from build123d import *

# Parameters (mm, degrees)
SKETCH10_W           = 35
SKETCH10_H           = 26
BOSS_EXTRUDE4_DEPTH  = 2.5
SKETCH1_R            = 1.5
BOSS_EXTRUDE5_DEPTH  = 5
SKETCH11_W           = 35
SKETCH11_H           = 26
BOSS_EXTRUDE6_DEPTH  = 2.5
CUT_EXTRUDE1_START   = -13
CUT_EXTRUDE1_DEPTH   = 56.676105727
SKETCH4_R            = 7.6
CUT_EXTRUDE2_DEPTH   = 1.2
SKETCH5_R            = 6.6
CUT_EXTRUDE3_DEPTH   = 50.27874954
SKETCH12_W           = 35
SKETCH12_H           = 26
BOSS_EXTRUDE7_DEPTH  = 15
SKETCH13_W           = 35
SKETCH13_H           = 26
BOSS_EXTRUDE8_DEPTH  = 7.5
SKETCH14_R           = 1.5
BOSS_EXTRUDE9_DEPTH  = 5
SKETCH15_W           = 35
SKETCH15_H           = 26
BOSS_EXTRUDE10_DEPTH = 2.5
SKETCH8_R            = 4
CUT_EXTRUDE6_DEPTH   = 62.021677757
FILLET1_R            = 13


with BuildPart() as part:
    # Sketch10 → Boss-Extrude4 (new body)
    with BuildSketch(Plane(origin=(0, 0, 0), x_dir=(1, 0, 0), z_dir=(0, 1, 0))):
        with Locations((15.5, -23)):
            Rectangle(SKETCH10_W, SKETCH10_H)
    extrude(amount=BOSS_EXTRUDE4_DEPTH)

    # Sketch1 → Boss-Extrude5 (add)
    with BuildSketch(Plane(origin=(0, 0, 0), x_dir=(1, 0, 0), z_dir=(0, 1, 0))):
        Polygon((0, 0), (6, 0), (6, -10), (25, -10), (25, 0), (31, 0), (31, -10), (33, -10), (33, -36), (-2, -36), (-2, -10), (0, -10), align=None)
        with Locations(Location((3, -5, 0), (0, 0, 270))):
            Circle(SKETCH1_R, mode=Mode.SUBTRACT)
        with Locations(Location((28, -5, 0), (0, 0, 90))):
            Circle(SKETCH1_R, mode=Mode.SUBTRACT)
    extrude(amount=-BOSS_EXTRUDE5_DEPTH)

    # Sketch11 → Boss-Extrude6 (add)
    with BuildSketch(Plane.XZ.offset(5)):
        with Locations((15.5, 23)):
            Rectangle(SKETCH11_W, SKETCH11_H)
    extrude(amount=BOSS_EXTRUDE6_DEPTH)

    # Sketch3 → Cut-Extrude1 (cut)
    with BuildSketch(Plane(origin=(0, 0, 10), x_dir=(-1, 0, 0), z_dir=(0, 0, -1)).offset(CUT_EXTRUDE1_START)):
        Polygon((-22.1, 2.5), (-22.1, 0.2875), (-23.1, 0.2875), (-23.1, -0.9125), (-15.5, -0.9125), (-7.9, -0.9125), (-7.9, 0.2875), (-8.9, 0.2875), (-8.9, 2.5), align=None)
    cut_extrude1 = extrude(amount=CUT_EXTRUDE1_DEPTH, mode=Mode.SUBTRACT)

    # Sketch4 → Cut-Extrude2 (cut)
    with BuildSketch(Plane(origin=(0, -0.9125, 0), x_dir=(1, 0, 0), z_dir=(0, 1, 0))):
        with Locations((15.5, -23)):
            Circle(SKETCH4_R)
    cut_extrude2 = extrude(amount=CUT_EXTRUDE2_DEPTH, mode=Mode.SUBTRACT)

    # Sketch5 → Cut-Extrude3 (cut, through all)
    with BuildSketch(Plane(origin=(0, -0.9125, 0), x_dir=(1, 0, 0), z_dir=(0, 1, 0))):
        with Locations((15.5, -23)):
            Circle(SKETCH5_R)
    cut_extrude3 = extrude(amount=CUT_EXTRUDE3_DEPTH, mode=Mode.SUBTRACT)

    # Sketch12 → Boss-Extrude7 (add)
    with BuildSketch(Plane.XZ.offset(7.5)):
        with Locations((15.5, 23)):
            Rectangle(SKETCH12_W, SKETCH12_H)
    extrude(amount=BOSS_EXTRUDE7_DEPTH)

    # Sketch13 → Boss-Extrude8 (add)
    with BuildSketch(Plane.XZ.offset(22.5)):
        with Locations((15.5, 23)):
            Rectangle(SKETCH13_W, SKETCH13_H)
    extrude(amount=BOSS_EXTRUDE8_DEPTH)

    # Sketch14 → Boss-Extrude9 (add)
    with BuildSketch(Plane.XZ.offset(30)):
        Polygon((0, 0), (6, 0), (6, 10), (25, 10), (25, 0), (31, 0), (31, 10), (33, 10), (33, 36), (-2, 36), (-2, 10), (0, 10), align=None)
        with Locations(Location((3, 5, 0), (0, 0, 90))):
            Circle(SKETCH14_R, mode=Mode.SUBTRACT)
        with Locations(Location((28, 5, 0), (0, 0, 270))):
            Circle(SKETCH14_R, mode=Mode.SUBTRACT)
    extrude(amount=BOSS_EXTRUDE9_DEPTH)

    # Sketch15 → Boss-Extrude10 (add)
    with BuildSketch(Plane.XZ.offset(35)):
        with Locations((15.5, 23)):
            Rectangle(SKETCH15_W, SKETCH15_H)
    extrude(amount=BOSS_EXTRUDE10_DEPTH)

    # Mirror8: Cut-Extrude1, Cut-Extrude2, Cut-Extrude3 across plane
    add(cut_extrude1.mirror(Plane.ZX.offset(-17.5)), mode=Mode.SUBTRACT)
    add(cut_extrude2.mirror(Plane.ZX.offset(-17.5)), mode=Mode.SUBTRACT)
    add(cut_extrude3.mirror(Plane.ZX.offset(-17.5)), mode=Mode.SUBTRACT)

    # Sketch8 → Cut-Extrude6 (cut, through all)
    with BuildSketch(Plane(origin=(0, -0.9125, 0), x_dir=(1, 0, 0), z_dir=(0, 1, 0))):
        with Locations(Location((15.5, -23, 0), (0, 0, 270))):
            Circle(SKETCH8_R)
    extrude(amount=-CUT_EXTRUDE6_DEPTH, mode=Mode.SUBTRACT)

    # Fillet1
    fillet1_edges = [part.edges().sort_by_distance(p)[0] for p in [
        (33, -17.5, 36),
        (-2, -17.5, 36),
    ]]
    fillet(fillet1_edges, radius=FILLET1_R)


solid = part.part
Design review of the part built by this model. Coordinates are the model's own, in mm. A direction names the side the tool comes from. Give positions to 0.01 mm unless a question says otherwise; leave off trailing zeros. Loops run counter-clockwise (first coordinate to the right, second up) from the corner with the lowest first, then second, coordinate; pieces in that order, holes last. Notation, with made-up numbers: (-1.5, 1.5) - (22.5, 1.5) arc R21 ccw to (22.5, 38.5) - close; hole circle Ø8 at (48.25, 56). An arc over 180 degrees is marked (long way). Use CSV: the item, a comma, the result in double quotes. Start each with the question number.
1. Wall thickness on L1, parallel to X at y = -32.15, z = 5; L2, parallel to Y at x = 23, z = 18; L3, parallel to X at y = 1, z = 17.5: over which ranges is each line inside the solid? List them lowest first.
2. Add section D-D (y = -8.5). State the section outline as (x, z) points, plus the area to 3 significant figures.
3. Machinability: for faces 5 (the flat face through (22.1, -36, 17)), 6 (the flat face through (25, -32, 5)), 7 (the flat face through (4.4, 0, 6)), which of the approach directions +Z, -Z, +X, -X, +Y, -Y give a long, thin tool a straight path to every point of the face, cutting with its end or side? Answer none if there is none.
4. Add section A-A (x = 15.5). State the section outline as (y, z) points, plus the area to 3 significant figures.
5. Add section B-B (z = 5). Count the separate pieces of the cut face and the enclosed holes in it, plus the area to 3 significant figures.
6. Add section C-C (y = -33). State the section outline as (x, z) points.
7. Draft analysis for pull direction Y (two halves, no side actions). For faces 1 (the flat face through (11, -37.5, 29)), 2 (the cylindrical face through (15.4, -36.4, 29.6)), 3 (the cylindrical face through (15.33, -0.32, 30.6)), 4 (the flat face through (8.7, -35.288, 21.1)), state which applies: released by +Y, released by -Y, zero draft, split by the parting line, or undercut.
8. Insertion check: P1, Ø3, axis at x = 3.5, y = -25.5, coming from the -Z side; P2, Ø4.5, axis at x = 17.5, z = 22, coming from the -Y side; P3, Ø12, axis at y = -26.5, z = 26.5, coming from the +X side; P4, Ø6.5, axis at x = 4.5, z = 5, coming from the +Y side. Each pin has a flat end and moves straight along its axis. Give the tip position at first contact, or say it passes through.
Results found:
1,L1,"x = 0 to 1.5, 4.5 to 6, 25 to 26.5, 29.5 to 31"
1,L2,"y = -37.5 to -35.29, -34.09 to -0.91, 0.29 to 2.5"
1,L3,"x = -2 to 8.9, 22.1 to 33"
2,outline,"(-2, 10) - (33, 10) - (33, 23) arc R13 ccw to (20, 36) - (11, 36) arc R13 ccw to (-2, 23) - close; hole circle Ø8 at (15.5, 23)"
2,area,"787 mm²"
3,face 5,"-Z, -Y"
3,face 6,"-Z, +Y, -Y"
3,face 7,"-Z, +X, -X, +Y"
4,outline,"(-37.5, 29.6) - (-35.29, 29.6) - (-35.29, 30.6) - (-34.09, 30.6) - (-34.09, 27) - (-0.91, 27) - (-0.91, 30.6) - (0.29, 30.6) - (0.29, 29.6) - (2.5, 29.6) - (2.5, 36) - (-37.5, 36) - close; (-34.09, 10) - (-0.91, 10) - (-0.91, 19) - (-34.09, 19) - close"
4,area,"638 mm²"
5,separate pieces,"8"
5,enclosed holes,"0"
5,area,"60.0 mm²"
6,outline,"(-2, 10) - (0, 10) - (0, 0) - (6, 0) - (6, 10) - (25, 10) - (25, 0) - (31, 0) - (31, 10) - (33, 10) - (33, 23) arc R13 ccw to (20, 36) - (11, 36) arc R13 ccw to (-2, 23) - close; hole circle Ø3 at (3, 5); hole circle Ø8 at (15.5, 23); hole circle Ø3 at (28, 5)"
7,face 1,"released by -Y"
7,face 2,"zero draft"
7,face 3,"undercut"
7,face 4,"undercut"
8,P1,"stops at z = 10"
8,P2,"stops at y = -34.09"
8,P3,"stops at x = 33"
8,P4,"stops at y = 0"
